```python
from build123d import *

# Parameters (mm, degrees)
CROQUIS1_R              = 10
SALIENTE_EXTRUIR1_DEPTH = 1
CROQUIS2_R              = 2
CROQUIS2_R_2            = 1.5
CORTAR_EXTRUIR1_DEPTH   = 1
CORTAR_EXTRUIR2_DEPTH   = 1
CORTAR_EXTRUIR3_DEPTH   = 1
CORTAR_EXTRUIR4_DEPTH   = 1


with BuildPart() as part:
    # Croquis1 → Saliente-Extruir1 (new body)
    with BuildSketch(Plane.XY):
        with BuildLine():
            Line((-35, -40), (35, -40))
            ThreePointArc((35, -40), (38.535533906, -38.535533906), (40, -35))
            Line((40, -35), (40, 35))
            ThreePointArc((40, 35), (38.535533906, 38.535533906), (35, 40))
            Line((35, 40), (-35, 40))
            ThreePointArc((-35, 40), (-38.535533906, 38.535533906), (-40, 35))
            Line((-40, 35), (-40, -35))
            ThreePointArc((-40, -35), (-38.535533906, -38.535533906), (-35, -40))
        make_face()
        Circle(CROQUIS1_R, mode=Mode.SUBTRACT)
    extrude(amount=-SALIENTE_EXTRUIR1_DEPTH)

    # Croquis2 → Cortar-Extruir1 (cut)
    with BuildSketch(Plane.XY):
        with Locations((36, 0)):
            Circle(CROQUIS2_R)
        with Locations(Location((-36, 0, 0), (0, 0, 180))):
            Circle(CROQUIS2_R)
        with Locations((32.5, -32.5)):
            Circle(CROQUIS2_R_2)
        with Locations(Location((32.5, 32.5, 0), (0, 0, 180))):
            Circle(CROQUIS2_R_2)
        with Locations(Location((-32.5, -32.5, 0), (0, 0, 180))):
            Circle(CROQUIS2_R_2)
        with Locations((-32.5, 32.5)):
            Circle(CROQUIS2_R_2)
        with Locations((10.7, -8.5)):
            Circle(CROQUIS2_R)
        with Locations(Location((-10.7, -8.5, 0), (0, 0, 180))):
            Circle(CROQUIS2_R)
    extrude(amount=-CORTAR_EXTRUIR1_DEPTH, mode=Mode.SUBTRACT)

    # Croquis3 → Cortar-Extruir2 (cut)
    with BuildSketch(Plane.XY):
        with BuildLine():
            Line((-7.8, 26.5), (7.8, 26.5))
            ThreePointArc((7.8, 26.5), (9.3, 28), (7.8, 29.5))
            Line((7.8, 29.5), (-7.8, 29.5))
            ThreePointArc((-7.8, 29.5), (-9.3, 28), (-7.8, 26.5))
        make_face()
        with BuildLine():
            Line((-7.8, 34.5), (7.8, 34.5))
            ThreePointArc((7.8, 34.5), (9.3, 33), (7.8, 31.5))
            Line((7.8, 31.5), (-7.8, 31.5))
            ThreePointArc((-7.8, 31.5), (-9.3, 33), (-7.8, 34.5))
        make_face()
        with BuildLine():
            Line((-7.8, 21.5), (7.8, 21.5))
            ThreePointArc((7.8, 21.5), (9.3, 23), (7.8, 24.5))
            Line((7.8, 24.5), (-7.8, 24.5))
            ThreePointArc((-7.8, 24.5), (-9.3, 23), (-7.8, 21.5))
        make_face()
        with BuildLine():
            Line((-7.8, 16.5), (7.8, 16.5))
            ThreePointArc((7.8, 16.5), (9.3, 18), (7.8, 19.5))
            Line((7.8, 19.5), (-7.8, 19.5))
            ThreePointArc((-7.8, 19.5), (-9.3, 18), (-7.8, 16.5))
        make_face()
        with BuildLine():
            Line((-7.8, 11.5), (7.8, 11.5))
            ThreePointArc((7.8, 11.5), (9.3, 13), (7.8, 14.5))
            Line((7.8, 14.5), (-7.8, 14.5))
            ThreePointArc((-7.8, 14.5), (-9.3, 13), (-7.8, 11.5))
        make_face()
        with BuildLine():
            Line((-10.95, -30), (10.95, -30))
            ThreePointArc((10.95, -30), (12.45, -28.5), (10.95, -27))
            Line((10.95, -27), (-10.95, -27))
            ThreePointArc((-10.95, -27), (-12.45, -28.5), (-10.95, -30))
        make_face()
        with BuildLine():
            Line((-10.95, -32), (10.95, -32))
            ThreePointArc((10.95, -32), (12.45, -33.5), (10.95, -35))
            Line((10.95, -35), (-10.95, -35))
            ThreePointArc((-10.95, -35), (-12.45, -33.5), (-10.95, -32))
        make_face()
        with BuildLine():
            Line((-10.95, -25), (10.95, -25))
            ThreePointArc((10.95, -25), (12.45, -23.5), (10.95, -22))
            Line((10.95, -22), (-10.95, -22))
            ThreePointArc((-10.95, -22), (-12.45, -23.5), (-10.95, -25))
        make_face()
        with BuildLine():
            Line((-10.95, -20), (10.95, -20))
            ThreePointArc((10.95, -20), (12.45, -18.5), (10.95, -17))
            Line((10.95, -17), (-10.95, -17))
            ThreePointArc((-10.95, -17), (-12.45, -18.5), (-10.95, -20))
        make_face()
        with BuildLine():
            Line((-10.95, -15), (10.95, -15))
            ThreePointArc((10.95, -15), (12.45, -13.5), (10.95, -12))
            Line((10.95, -12), (-10.95, -12))
            ThreePointArc((-10.95, -12), (-12.45, -13.5), (-10.95, -15))
        make_face()
    extrude(amount=-CORTAR_EXTRUIR2_DEPTH, mode=Mode.SUBTRACT)

    # Croquis4 → Cortar-Extruir3 (cut)
    with BuildSketch(Plane.XY):
        with BuildLine():
            Line((11, 2.7), (11, 33))
            ThreePointArc((11, 33), (12.5, 34.5), (14, 33))
            Line((14, 33), (14, 2.7))
            ThreePointArc((14, 2.7), (12.5, 1.2), (11, 2.7))
        make_face()
        with BuildLine():
            Line((17, 2.7), (17, 33))
            ThreePointArc((17, 33), (18.5, 34.5), (20, 33))
            Line((20, 33), (20, 2.7))
            ThreePointArc((20, 2.7), (18.5, 1.2), (17, 2.7))
        make_face()
        with BuildLine():
            Line((23, 2.7), (23, 33))
            ThreePointArc((23, 33), (24.5, 34.5), (26, 33))
            Line((26, 33), (26, 2.7))
            ThreePointArc((26, 2.7), (24.5, 1.2), (23, 2.7))
        make_face()
        with BuildLine():
            Line((32, 25.9), (32, 2.7))
            ThreePointArc((32, 2.7), (30.5, 1.2), (29, 2.7))
            Line((29, 2.7), (29, 25.9))
            ThreePointArc((29, 25.9), (30.5, 27.4), (32, 25.9))
        make_face()
        with BuildLine():
            Line((-11, 2.7), (-11, 33))
            ThreePointArc((-11, 33), (-12.5, 34.5), (-14, 33))
            Line((-14, 33), (-14, 2.7))
            ThreePointArc((-14, 2.7), (-12.5, 1.2), (-11, 2.7))
        make_face()
        with BuildLine():
            Line((-17, 2.7), (-17, 33))
            ThreePointArc((-17, 33), (-18.5, 34.5), (-20, 33))
            Line((-20, 33), (-20, 2.7))
            ThreePointArc((-20, 2.7), (-18.5, 1.2), (-17, 2.7))
        make_face()
        with BuildLine():
            Line((-23, 2.7), (-23, 33))
            ThreePointArc((-23, 33), (-24.5, 34.5), (-26, 33))
            Line((-26, 33), (-26, 2.7))
            ThreePointArc((-26, 2.7), (-24.5, 1.2), (-23, 2.7))
        make_face()
        with BuildLine():
            Line((-32, 25.9), (-32, 2.7))
            ThreePointArc((-32, 2.7), (-30.5, 1.2), (-29, 2.7))
            Line((-29, 2.7), (-29, 25.9))
            ThreePointArc((-29, 25.9), (-30.5, 27.4), (-32, 25.9))
        make_face()
    extrude(amount=-CORTAR_EXTRUIR3_DEPTH, mode=Mode.SUBTRACT)

    # Croquis5 → Cortar-Extruir4 (cut)
    with BuildSketch(Plane.XY):
        with BuildLine():
            Line((17, -3.5), (17, -33.5))
            ThreePointArc((17, -33.5), (15.5, -35), (14, -33.5))
            Line((14, -33.5), (14, -3.5))
            ThreePointArc((14, -3.5), (15.5, -2), (17, -3.5))
        make_face()
        with BuildLine():
            Line((20, -3.5), (20, -33.5))
            ThreePointArc((20, -33.5), (21.5, -35), (23, -33.5))
            Line((23, -33.5), (23, -3.5))
            ThreePointArc((23, -3.5), (21.5, -2), (20, -3.5))
        make_face()
        with BuildLine():
            Line((29, -3.5), (29, -27))
            ThreePointArc((29, -27), (27.5, -28.5), (26, -27))
            Line((26, -27), (26, -3.5))
            ThreePointArc((26, -3.5), (27.5, -2), (29, -3.5))
        make_face()
        with BuildLine():
            Line((32, -27), (32, -6))
            ThreePointArc((32, -6), (33.5, -4.5), (35, -6))
            Line((35, -6), (35, -27))
            ThreePointArc((35, -27), (33.5, -28.5), (32, -27))
        make_face()
        with BuildLine():
            Line((-17, -3.5), (-17, -33.5))
            ThreePointArc((-17, -33.5), (-15.5, -35), (-14, -33.5))
            Line((-14, -33.5), (-14, -3.5))
            ThreePointArc((-14, -3.5), (-15.5, -2), (-17, -3.5))
        make_face()
        with BuildLine():
            Line((-23, -3.5), (-23, -33.5))
            ThreePointArc((-23, -33.5), (-21.5, -35), (-20, -33.5))
            Line((-20, -33.5), (-20, -3.5))
            ThreePointArc((-20, -3.5), (-21.5, -2), (-23, -3.5))
        make_face()
        with BuildLine():
            Line((-29, -3.5), (-29, -27))
            ThreePointArc((-29, -27), (-27.5, -28.5), (-26, -27))
            Line((-26, -27), (-26, -3.5))
            ThreePointArc((-26, -3.5), (-27.5, -2), (-29, -3.5))
        make_face()
        with BuildLine():
            Line((-32, -27), (-32, -6))
            ThreePointArc((-32, -6), (-33.5, -4.5), (-35, -6))
            Line((-35, -6), (-35, -27))
            ThreePointArc((-35, -27), (-33.5, -28.5), (-32, -27))
        make_face()
    extrude(amount=-CORTAR_EXTRUIR4_DEPTH, mode=Mode.SUBTRACT)


solid = part.part
```
The model under review builds one solid part; all positions refer to its coordinate system, in mm. Round coordinates to 2 decimals unless told otherwise and drop trailing zeros. Write each loop counter-clockwise with the first axis right and the second up, starting at its lowest first coordinate (ties: lowest second). Pieces come first, ordered by that corner, then holes.
(1) We need section A-A on x = 24.5. Give the boundary of the cut face in (y, z), and give its area (3 significant figures).
(2) Insertion check: pin 1 (1.8 mm diameter, centred on x = -32.5, y = -32.5, fed in from -Z); pin 2 (3 mm diameter, centred on x = 31, y = -25, fed in from +Z). Each pin has a flat end and moves straight along its axis. Give the tip position at first contact, or say it passes through.
(3) We need section B-B on y = -18.5. Give the number of separate pieces and of enclosed holes in the cut face, and give its area (3 significant figures).
(4) We need section D-D on x = 15.5. Give the boundary of the cut face in (y, z), and give its area (3 significant figures).
(5) Mouldability with a two-part tool opening along Y and no side actions: class faces 1 (the flat face through (-9, 9, -1)), 2 (the cylindrical face through (-10.44, -10.483, -0.493)), 3 (the cylindrical face through (37.847, -0.766, -0.493)), 4 (the cylindrical face through (38.57, 38.5, -0.49)) as +Y half, -Y half, draft (parallel to the pull), parting line (faces both ways), or undercut.
(6) Wall thickness on L1, parallel to Y at x = -32.5, z = -0.5; L2, parallel to X at y = -1, z = -0.1; L3, parallel to Y at x = -16.5, z = -0.8: over which ranges is each line inside the solid? List them lowest first.
Findings below:
1. outline: (-40, -1) - (1.2, -1) - (1.2, 0) - (-40, 0) - close; (34.5, -1) - (40, -1) - (40, 0) - (34.5, 0) - close
1. area: 46.7 mm2
2. pin 1: passes through
2. pin 2: stops at z = 0
3. separate pieces: 10
3. enclosed holes: 0
3. area: 31.1 mm2
4. outline: (-40, -1) - (-35, -1) - (-35, 0) - (-40, 0) - close; (-2, -1) - (40, -1) - (40, 0) - (-2, 0) - close
4. area: 47.0 mm2
5. face 1: draft
5. face 2: undercut
5. face 3: undercut
5. face 4: +Y half
6. L1: y = -40 to -34, -31 to -28.12, -4.88 to 31, 34 to 40
6. L2: x = -40 to -37.73, -34.27 to -9.95, 9.95 to 34.27, 37.73 to 40
6. L3: y = -40 to -34.62, -2.38 to 40
